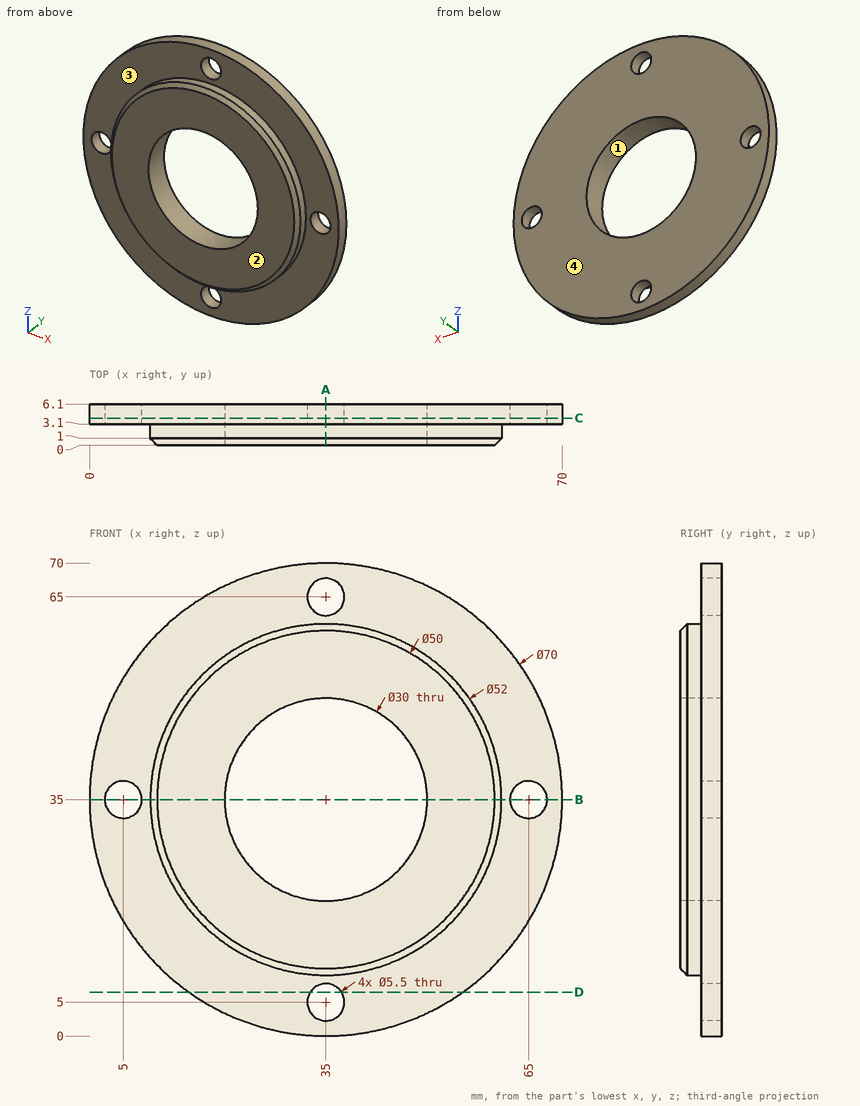
Answer from the drawing. Dimensions are ordinates in mm from the lowest x, y and z of the part. A direction names the side the tool comes from. Give positions to 0.01 mm unless a question says otherwise; leave off trailing zeros. Loops run counter-clockwise (first coordinate to the right, second up) from the corner with the lowest first, then second, coordinate; pieces in that order, holes last. Notation, with made-up numbers: (0, 13.25) -> (9, 13.25) arc R10 cw to (9, 19.25) -> close; hole circle Ø2 at (-25, -22.5). An arc over 180 degrees is marked (long way). Use a Markdown table: item, result.
Q1. Section C-C, the plane y = 4 is taken. Determine the outline of the cut face in (x, z), then the cut area to 3 significant figures.
Solved:
| item | result |
|---|---|
| outline | circle Ø70 at (35, 35); hole circle Ø5.5 at (5, 35); hole circle Ø30 at (35, 35); hole circle Ø5.5 at (35, 5); hole circle Ø5.5 at (35, 65); hole circle Ø5.5 at (65, 35) |
| area | 3,050 mm^2 |
Q2. A tool of negligible diameter and unlimited length cuts with its end or side. For the marked faces 3 and 4, from which of +Z, -Z, +X, -X, +Y, -Y can it reach the whole face along a straight path? Write none if from no direction.
Solved:
| item | result |
|---|---|
| face 3 | -Y |
| face 4 | +Z, -Z, +X, -X, +Y |
Q3. Section B-B, the plane z = 35 is taken. Determine the outline of the cut face in (x, y), then the cut area to 3 significant figures.
Solved:
| item | result |
|---|---|
| outline | (0, 3.1) -> (2.25, 3.1) -> (2.25, 6.1) -> (0, 6.1) -> close; (7.75, 3.1) -> (9, 3.1) -> (9, 1) -> (10, 0) -> (20, 0) -> (20, 6.1) -> (7.75, 6.1) -> close; (50, 0) -> (60, 0) -> (61, 1) -> (61, 3.1) -> (62.25, 3.1) -> (62.25, 6.1) -> (50, 6.1) -> close; (67.75, 3.1) -> (70, 3.1) -> (70, 6.1) -> (67.75, 6.1) -> close |
| area | 154 mm^2 |
Q4. Determine the mould class of the marked faces 1 and 2 for opening direction Z: pulls with the +Z half, pulls with the -Z half, needs draft (parallel to the pull), parting line crosses it, or undercut.
Solved:
| item | result |
|---|---|
| face 1 | undercut |
| face 2 | needs draft |
Q5. Each of these flat-tipped pins is pushed along its axis until it touches: pin 1 (3 mm diameter, centred on y = 1.5, z = 54.5, fed in from +X); pin 2 (2 mm diameter, centred on x = 44.5, y = 4, fed in from -Z); pin 3 (3 mm diameter, centred on y = 1, z = 55, fed in from +X). Where does it stop, or does it pass through?
Solved:
| item | result |
|---|---|
| pin 1 | stops at x = 53.76 |
| pin 2 | stops at z = 1.05 |
| pin 3 | stops at x = 53.27 |
Q6. Section A-A, the plane x = 35 is taken. Determine the outline of the cut face in (y, z), then the cut area to 3 significant figures.
Solved:
| item | result |
|---|---|
| outline | (0, 10) -> (1, 9) -> (3.1, 9) -> (3.1, 7.75) -> (6.1, 7.75) -> (6.1, 20) -> (0, 20) -> close; (0, 50) -> (6.1, 50) -> (6.1, 62.25) -> (3.1, 62.25) -> (3.1, 61) -> (1, 61) -> (0, 60) -> close; (3.1, 0) -> (6.1, 0) -> (6.1, 2.25) -> (3.1, 2.25) -> close; (3.1, 67.75) -> (6.1, 67.75) -> (6.1, 70) -> (3.1, 70) -> close |
| area | 154 mm^2 |
Q7. Section D-D, the plane z = 6.5 is taken. Determine the outline of the cut face in (x, y), then the cut area to 3 significant figures.
Solved:
| item | result |
|---|---|
| outline | (14.68, 3.1) -> (32.7, 3.1) -> (32.7, 6.1) -> (14.68, 6.1) -> close; (37.3, 3.1) -> (55.32, 3.1) -> (55.32, 6.1) -> (37.3, 6.1) -> close |
| area | 108 mm^2 |
Q8. Find the intervals of material crossed by line 1 along Z through (x, y) = (35, 5); line 2 along X through (y, z) = (3, 48); line 3 along Y through (x, z) = (64.5, 49.5), in increasing order.
Solved:
| item | result |
|---|---|
| line 1 | z = 0 to 2.25, 7.75 to 20, 50 to 62.25, 67.75 to 70 |
| line 2 | x = 12.48 to 27.52, 42.48 to 57.52 |
| line 3 | y = 3.1 to 6.1 |
